Could you check a few things on this model? Use its own coordinates, in mm. A direction names the side the tool comes from. Round coordinates to 2 decimals unless told otherwise and drop trailing zeros. Loops run counter-clockwise (first coordinate to the right, second up) from the corner with the lowest first, then second, coordinate; pieces in that order, holes last. Notation, with made-up numbers: (-18, -29) -> (-5, -29) arc R15 cw to (-5, 0) -> close; hole circle Ø10 at (87.5, 14.5). An arc over 180 degrees is marked (long way). Use CSV: the item, a comma, the result in double quotes. Start each with the question number.
```python
from build123d import *

# Parameters (mm, degrees)
SKETCH1_R           = 16
BOSS_EXTRUDE1_DEPTH = 5
SKETCH3_R           = 15
CUT_EXTRUDE1_DEPTH  = 4
FILLET1_R           = 0.5
SKETCH7_W           = 5.268501054
SKETCH7_H           = 14.735182388
CUT_EXTRUDE2_DEPTH  = 11
SKETCH8_R           = 7.4
BOSS_EXTRUDE2_DEPTH = 4
SKETCH9_R           = 3.45
CUT_EXTRUDE3_DEPTH  = 1
SKETCH11_R          = 1.969447503
CUT_EXTRUDE4_DEPTH  = 10


with BuildPart() as part:
    # Sketch1 → Boss-Extrude1 (new body)
    with BuildSketch(Plane.XY):
        Circle(SKETCH1_R)
    extrude(amount=BOSS_EXTRUDE1_DEPTH)

    # Sketch3 → Cut-Extrude1 (cut)
    with BuildSketch(Plane.XY.offset(5)):
        Circle(SKETCH3_R)
    extrude(amount=-CUT_EXTRUDE1_DEPTH, mode=Mode.SUBTRACT)

    # Fillet1
    fillet1_edges = [part.edges().sort_by_distance(p)[0] for p in [
        (-15, 0, 1),
    ]]
    fillet(fillet1_edges, radius=FILLET1_R)

    # Sketch7 → Cut-Extrude2 (cut)
    with BuildSketch(Plane.XY.offset(13)):
        with Locations((-14.456252894, -1.028256592)):
            Rectangle(SKETCH7_W, SKETCH7_H)
    cut_extrude2 = extrude(amount=-CUT_EXTRUDE2_DEPTH, mode=Mode.SUBTRACT)

    # Mirror1: Cut-Extrude2 across plane
    add(cut_extrude2.mirror(Plane(origin=(0, 0, 0), x_dir=(0, 0, 1), z_dir=(1, 0, 0))), mode=Mode.SUBTRACT)

    # Sketch8 → Boss-Extrude2 (add)
    with BuildSketch(Plane.XY.offset(1)):
        Circle(SKETCH8_R)
    extrude(amount=BOSS_EXTRUDE2_DEPTH)

    # Sketch9 → Cut-Extrude3 (cut)
    with BuildSketch(Plane.XY.offset(5)):
        Circle(SKETCH9_R)
    extrude(amount=-CUT_EXTRUDE3_DEPTH, mode=Mode.SUBTRACT)

    # Sketch11 → Cut-Extrude4 (cut)
    with BuildSketch(Plane.XY.offset(5)):
        with Locations((-5.549660814, 0)):
            Circle(SKETCH11_R)
    extrude(amount=-CUT_EXTRUDE4_DEPTH, mode=Mode.SUBTRACT)


solid = part.part
```
1. Suppose I cut it at B-B (z = 4.6). List the corners of the cut face in (x, y) for me, then the cut area to 3 significant figures.
2. If I drill on L1, parallel to Y at x = 0, z = 2.5; L2, parallel to Y at x = -4, z = 2.55; L3, parallel to Y at x = -1.5, z = 1.5, over which ranges is the centre line in solid material (lowest first)?
3. For faces 4 (the face through (-0.45, 3.42, 4.51)), 5 (the face through (-0.1, -15.3, 5)), 6 (the face through (13, -8.396, 4)), which set-ups out of +Z, -Z, +X, -X, +Y, -Y let a thin tool reach every point of the face, with its end or its side?
4. Will these pins go through, and if not, where does the flat tip stop? pin 1 (1.3 mm diameter, centred on x = 13, z = 3, fed in from +Y); pin 2 (4 mm diameter, centred on x = 13.5, y = 2, fed in from +Z); pin 3 (1 mm diameter, centred on x = 3, z = 2.5, fed in from -Y); pin 4 (3.5 mm diameter, centred on x = -5.55, y = 0, fed in from +Z).
5. Suppose I cut it at A-A (x = 0). List the corners of the cut face in (y, z) for me.
6. We'd pull the mould along X, two halves only. Please class faces 1 (the face through (0, 0, 4)), 2 (the face through (-15.15, -0.99, 2)), 3 (the face through (-15.985, 0.703, 1.354)): pulls with the +X half, pulls with the -X half, needs draft (parallel to the pull), parting line crosses it, or undercut.
Geometry check:
1,outline,"(-14.69, 6.34) -> (-13.59, 6.34) arc R15 cw to (13.59, 6.34) -> (14.69, 6.34) arc R16 ccw to start; (-13.62, -8.4) arc R16 ccw to (13.62, -8.4) -> (12.43, -8.4) arc R15 cw to (-12.43, -8.4) -> close; (-7.36, -0.78) arc R7.4 ccw (long way) to (-7.36, 0.78) arc R1.97 cw (long way) to start; hole circle Ø6.9 at (0, 0)"
1,area,"189 mm²"
2,L1,"y = -16 to -15, -7.4 to 7.4, 15 to 16"
2,L2,"y = -15.49 to -14.46, -6.23 to -1.22, 1.22 to 6.23, 14.46 to 15.49"
2,L3,"y = -15.93 to -14.92, -7.25 to 7.25, 14.92 to 15.93"
3,face 4,"+Z"
3,face 5,"+Z, +X, -X, +Y, -Y"
3,face 6,"+Z, +X, -X"
4,pin 1,"stops at y = 10.17"
4,pin 2,"stops at z = 2"
4,pin 3,"stops at y = -15.8"
4,pin 4,"passes through"
5,outline,"(-16, 0) -> (16, 0) -> (16, 5) -> (15, 5) -> (15, 1.5) arc R0.5 cw to (14.5, 1) -> (7.4, 1) -> (7.4, 5) -> (3.45, 5) -> (3.45, 4) -> (-3.45, 4) -> (-3.45, 5) -> (-7.4, 5) -> (-7.4, 1) -> (-14.5, 1) arc R0.5 cw to (-15, 1.5) -> (-15, 5) -> (-16, 5) -> close"
6,face 1,"undercut"
6,face 2,"needs draft"
6,face 3,"parting line crosses it"
